Work out the finished part from the listing and answer in its coordinate system (mm). Face numbers are marked on the shaded views. A direction names the side the tool comes from. Coordinates: 2 decimals unless noted, no trailing zeros. Order: outer loops, then holes, each group sorted by start corner. A loop starts at its lowest first (then second) coordinate and runs counter-clockwise, first axis right, second up.
```python
from build123d import *

# Parameters (mm, degrees)
SKETCH1_W                = 2.625
SKETCH1_H                = 31.5
SKETCH1_W_2              = 7.5
SKETCH1_H_2              = 1.5
BOSS_EXTRUDE1_DEPTH      = 1.5
BOSS_EXTRUDE2_START      = 1.5
SKETCH1_3_W              = 7.5
SKETCH1_3_H              = 3
BOSS_EXTRUDE2_DEPTH      = 2
BOSS_EXTRUDE3_DEPTH      = 4
BOSS_EXTRUDE3_DEPTH_BACK = 3
BOSS_EXTRUDE3_START      = 1.5
SKETCH1_4_W              = 2.625
SKETCH1_4_H              = 31.5


with BuildPart() as part:
    # Sketch1 → Boss-Extrude1 (new body)
    with BuildSketch(Plane(origin=(0, 0, 0), x_dir=(1, 0, 0), z_dir=(0, 1, 0))):
        Polygon((-6.375, 15), (-6.375, -16.5), (6.375, -16.5), (6.375, 15), (9, 15), (9, 16.5), (3.75, 16.5), (3.75, 15), (-3.75, 15), (-3.75, 16.5), (-9, 16.5), (-9, 15), align=None)
        with Locations((-7.6875, -0.75)):
            Rectangle(SKETCH1_W, SKETCH1_H)
        with Locations((7.6875, -0.75)):
            Rectangle(SKETCH1_W, SKETCH1_H)
        with Locations((0, 15.75)):
            Rectangle(SKETCH1_W_2, SKETCH1_H_2)
    extrude(amount=BOSS_EXTRUDE1_DEPTH)

    # Sketch1<3> → Boss-Extrude2 (add)
    with BuildSketch(Plane(origin=(0, 0, 0), x_dir=(1, 0, 0), z_dir=(0, 1, 0)).offset(BOSS_EXTRUDE2_START)):
        with Locations((0, 16.5)):
            Rectangle(SKETCH1_3_W, SKETCH1_3_H)
    extrude(amount=BOSS_EXTRUDE2_DEPTH)

    # Sketch1<4> → Boss-Extrude3 (add, two sides: drawn at the far end of the back side and taken through both)
    with BuildSketch(Plane(origin=(0, 0, 0), x_dir=(1, 0, 0), z_dir=(0, 1, 0)).offset(BOSS_EXTRUDE3_START - BOSS_EXTRUDE3_DEPTH_BACK)):
        with Locations((-7.6875, -0.75)):
            Rectangle(SKETCH1_4_W, SKETCH1_4_H)
        with Locations((7.6875, -0.75)):
            Rectangle(SKETCH1_4_W, SKETCH1_4_H)
    extrude(amount=BOSS_EXTRUDE3_DEPTH + BOSS_EXTRUDE3_DEPTH_BACK)


solid = part.part
```
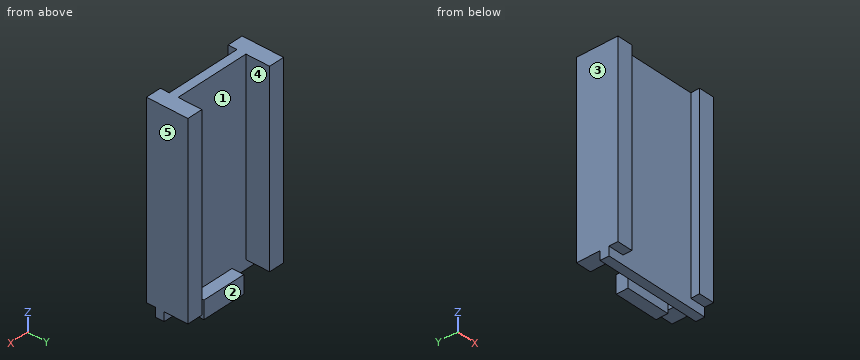
1. The mould has two halves that part along X. Classify the marked faces 1, 2 and 3: released by +X, released by -X, zero draft, split by the parting line, or undercut.
2. Flat-ended cylindrical pins translate along their axes: pin 1 (3 mm diameter, centred on x = 7, y = 4.5, fed in from -Z); pin 2 (2 mm diameter, centred on x = -0.5, y = 3, fed in from +Z); pin 3 (1.5 mm diameter, centred on x = 1.5, y = 0.5, fed in from -Z). Find the tip coordinate at first contact, or state that the pin passes through.
3. For the marked faces 4 and 5, determine the directions among +Z, -Z, +X, -X, +Y, -Y from which every point of the face is accessible in a straight line to the end or side of a thin tool.
4. The part is cut by section C-C (x = 2.75). Determine the outline of the cut face in (y, z).
5. The part is cut by section A-A (y = 2). Determine the outline of the cut face in (x, z) (3 decimals), plus the area to 3 significant figures.
6. Consider probe 1 along X at (y, z) = (3.25, 4.5) (3 decimals); probe 2 along Z at (x, y) = (-3.5, 2); probe 3 along Y at (x, z) = (1, -15.5). Determine where each line is inside the solid, lowest interval first.
7. The part is cut by section D-D (z = 5). Determine the outline of the cut face in (x, y) (3 decimals), plus the area to 3 significant figures.
8. The part is cut by section B-B (y = -0.5). Determine the outline of the cut face in (x, z) (3 decimals), plus the area to 3 significant figures.
Worked out:
1. face 1: undercut
1. face 2: zero draft
1. face 3: released by -X
2. pin 1: stops at z = -15
2. pin 2: stops at z = -15
2. pin 3: stops at z = -16.5
3. face 4: +Z, -Z, +Y
3. face 5: +Z, -Z, +X, +Y, -Y
4. outline: (0, -16.5) - (1.5, -16.5) - (1.5, -18) - (3.5, -18) - (3.5, -15) - (1.5, -15) - (1.5, 16.5) - (0, 16.5) - close
5. outline: (-9, -15) - (-6.375, -15) - (-6.375, 16.5) - (-9, 16.5) - close; (-3.75, -18) - (3.75, -18) - (3.75, -15) - (-3.75, -15) - close; (6.375, -15) - (9, -15) - (9, 16.5) - (6.375, 16.5) - close
5. area: 188 mm2
6. probe 1: x = -9 to -6.375, 6.375 to 9
6. probe 2: z = -18 to -15
6. probe 3: y = 0 to 3.5
7. outline: (-9, -1.5) - (-6.375, -1.5) - (-6.375, 0) - (6.375, 0) - (6.375, -1.5) - (9, -1.5) - (9, 5.5) - (6.375, 5.5) - (6.375, 1.5) - (-6.375, 1.5) - (-6.375, 5.5) - (-9, 5.5) - close
7. area: 55.9 mm2
8. outline: (-9, -15) - (-6.375, -15) - (-6.375, 16.5) - (-9, 16.5) - close; (6.375, -15) - (9, -15) - (9, 16.5) - (6.375, 16.5) - close
8. area: 165 mm2
